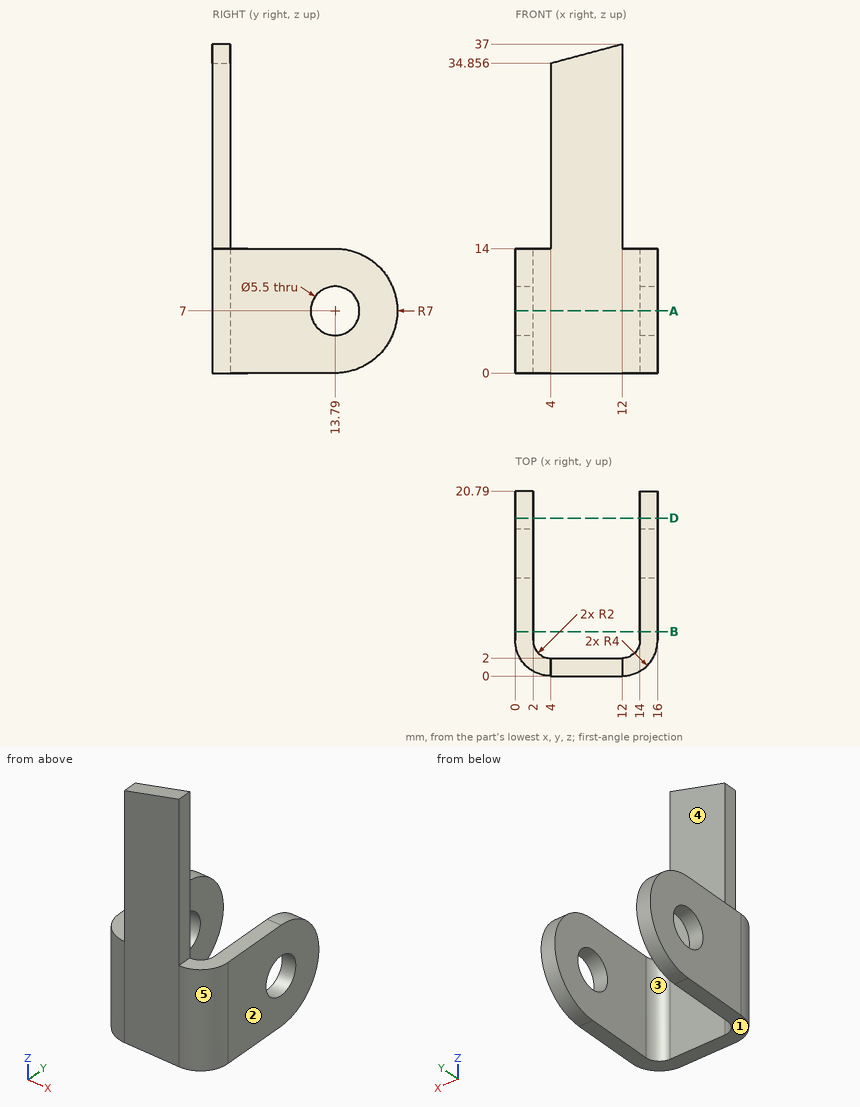
Print and shaded views of the part. All mm, measured from the part's lowest x, y and z. A direction names the side the tool comes from. Round coordinates to 2 decimals unless told otherwise and drop trailing zeros. Write each loop counter-clockwise with the first axis right and the second up, starting at its lowest first coordinate (ties: lowest second). Pieces come first, ordered by that corner, then holes. Notation, with made-up numbers: (85, 56.5) - (117, 56.5) arc R23 cw to (117, 92.5) - close; hole circle Ø8 at (-26, 26.25). An arc over 180 degrees is marked (long way). Write each question's results on one line, items separated by ' | '. Start each with the question number.
Item 1: Saw through at B-B (y = 5). Write the cut outline in (x, z).
Item 2: Saw through at A-A (z = 7). Write the cut outline in (x, y).
Item 3: Mould opens along X. For the marked faces 1, 2 and 3 say: pulls with the +X half, pulls with the -X half, needs draft (parallel to the pull), parting line crosses it, or undercut.
Item 4: Drop flat-ended pins along their axis: P1, Ø10, axis at y = 3, z = 28.5, coming from the -X side; P2, Ø5, axis at y = 13, z = 10.5, coming from the -X side; P3, Ø4.5, axis at x = 1.5, y = 8, coming from the +Z side; P4, Ø4, axis at x = 7.5, z = 22.5, coming from the +Y side. Give the stop position or say it passes through.
Item 5: Which spindle directions (+Z, -Z, +X, -X, +Y, -Y) get a long thin tool onto all of the face, cutting with end or side? Do the marked faces 4 and 5. Say none if no direction does.
Item 6: Saw through at D-D (y = 17.75). Write the cut outline in (x, z).
Item 7: Wall check: L1, parallel to X at y = 6.75, z = 5; L2, parallel to Y at x = 6.25, z = 27.5; L3, parallel to Y at x = 15, z = 7 (1 decimal). Give the ranges that are in metal, low to high. Write a range as [from, to].
Results are:
1) outline: (0, 0) - (2, 0) - (2, 14) - (0, 14) - close; (14, 0) - (16, 0) - (16, 14) - (14, 14) - close
2) outline: (0, 4) arc R4 ccw to (4, 0) - (12, 0) arc R4 ccw to (16, 4) - (16, 11.04) - (14, 11.04) - (14, 4) arc R2 cw to (12, 2) - (4, 2) arc R2 cw to (2, 4) - (2, 11.04) - (0, 11.04) - close; (0, 16.54) - (2, 16.54) - (2, 20.79) - (0, 20.79) - close; (14, 16.54) - (16, 16.54) - (16, 20.79) - (14, 20.79) - close
3) face 1: needs draft | face 2: pulls with the +X half | face 3: undercut
4) P1: stops at x = 4 | P2: stops at x = 0 | P3: stops at z = 14 | P4: stops at y = 2
5) face 4: +Z, -Z, +Y | face 5: +Z, -Z, +X, -Y
6) outline: (0, 1.23) - (2, 1.23) - (2, 12.77) - (0, 12.77) - close; (14, 1.23) - (16, 1.23) - (16, 12.77) - (14, 12.77) - close
7) L1: x = [0, 2], [14, 16] | L2: y = [0, 2] | L3: y = [1.4, 11], [16.5, 20.8]
